Input: part model. Units: mm. Frame: model coordinates. A direction names the side the tool comes from. Give positions to 0.01 mm unless a question says otherwise; leave off trailing zeros. Loops run counter-clockwise (first coordinate to the right, second up) from the corner with the lowest first, then second, coordinate; pieces in that order, holes last. Notation, with made-up numbers: (77, 39.25) -> (103, 39.25) arc R33 ccw to (103, 73.25) -> close; hole circle Ø9 at (24, 42.25). An arc over 180 degrees is marked (long way). Answer in a Markdown table with one row per item. Add a question column.
```python
from build123d import *

# Parameters (mm, degrees)
F0_W     = 32
F0_H     = 55
F3_DEPTH = 5
F1_R     = 1.75
F4_DEPTH = 19
F5_DEPTH = 5
F6_W     = 50
F6_H     = 4
F7_DEPTH = 1.8
F8_R     = 5
F9_R     = 5
F10_R    = 5
F11_R    = 5
F12_R    = 2
F13_R    = 1


with BuildPart() as f3:
    # F0 (on Front) → F3 (new body)
    with BuildSketch(Plane.XZ):
        with Locations((-113.3904078007, -8.5524536016)):
            Rectangle(F0_W, F0_H)
    extrude(amount=F3_DEPTH)

    # F1 (on face) → F4 (join)
    with BuildSketch(Plane.XZ):
        with Locations((-123.8904078007, 12.9475463984)):
            Circle(F1_R)
        with Locations((-102.8904078007, 12.9475463984)):
            Circle(F1_R)
    extrude(amount=F4_DEPTH)

    # F2 (on face) → F5 (cut)
    with BuildSketch(Plane.XZ):
        with BuildLine():
            ThreePointArc((-116.3904078007, -12.0524536016), (-113.3904078007, -15.0524536016), (-110.3904078007, -12.0524536016))
            ThreePointArc((-110.3904078007, -12.0524536016), (-113.3904078007, -9.0524536016), (-116.3904078007, -12.0524536016))
        make_face()
        with BuildLine():
            Line((-110.3904078007, -30.0524536016), (-110.3904078007, -12.0524536016))
            ThreePointArc((-110.3904078007, -12.0524536016), (-113.3904078007, -15.0524536016), (-116.3904078007, -12.0524536016))
            Line((-116.3904078007, -12.0524536016), (-116.3904078007, -30.0524536016))
            ThreePointArc((-116.3904078007, -30.0524536016), (-113.3904078007, -27.0524536016), (-110.3904078007, -30.0524536016))
        make_face()
        with BuildLine():
            ThreePointArc((-116.3904078007, -30.0524536016), (-113.3904078007, -33.0524536016), (-110.3904078007, -30.0524536016))
            ThreePointArc((-110.3904078007, -30.0524536016), (-113.3904078007, -27.0524536016), (-116.3904078007, -30.0524536016))
        make_face()
    extrude(amount=F5_DEPTH, mode=Mode.SUBTRACT)

    # F6 (on Front) → F7 (cut)
    with BuildSketch(Plane.XZ):
        with Locations((-109.2482896921, 6.9475463984)):
            Rectangle(F6_W, F6_H)
    extrude(amount=F7_DEPTH, mode=Mode.SUBTRACT)

    # F8
    f8_edges = [f3.edges().sort_by_distance(p)[0] for p in [
        (-97.390408, -2.5, 18.947546),
    ]]
    fillet(f8_edges, radius=F8_R)

    # F9
    f9_edges = [f3.edges().sort_by_distance(p)[0] for p in [
        (-129.390408, -2.5, 18.947546),
    ]]
    fillet(f9_edges, radius=F9_R)

    # F10
    f10_edges = [f3.edges().sort_by_distance(p)[0] for p in [
        (-129.390408, -2.5, -36.052454),
    ]]
    fillet(f10_edges, radius=F10_R)

    # F11
    f11_edges = [f3.edges().sort_by_distance(p)[0] for p in [
        (-97.390408, -2.5, -36.052454),
    ]]
    fillet(f11_edges, radius=F11_R)

    # F12
    f12_edges = [f3.edges().sort_by_distance(p)[0] for p in [
        (-98.854874, -5, 17.48308),
        (-113.390408, -5, 18.947546),
        (-127.925942, -5, 17.48308),
        (-129.390408, -5, -8.552454),
        (-127.925942, -5, -34.587988),
        (-113.390408, -5, -36.052454),
        (-97.390408, -5, -8.552454),
    ]]
    fillet(f12_edges, radius=F12_R)

    # F13
    f13_edges = [f3.edges().sort_by_distance(p)[0] for p in [
        (-125.640408, -19, 12.947546),
        (-104.640408, -19, 12.947546),
    ]]
    fillet(f13_edges, radius=F13_R)


solid = f3.part
```
1) Pull-direction query (Z, two-part tool) for faces 1 (the face through (-114, -1, 4.948)), 2 (the face through (-101.22, -11.41, 13.47)), 3 (the face through (-127.965, -1.521, -34.549)), 4 (the face through (-127.89, -1.52, 17.52)); classes: +Z half, -Z half, draft (parallel to the pull), parting line (faces both ways), or undercut.
2) Section A-A on z = -19.5. Output: boundary loops of the cut face in (x, y), and give its area (3 significant figures).
3) Section D-D on y = -4. Output: boundary loops of the cut face in (x, z).
4) Material intervals for line 1 along Z through (x, y) = (-112.5, -0.75); line 2 along Y through (x, z) = (-111.5, 3); line 3 along Y through (x, z) = (-107, 5.5), sorted ascending.
5) Section C-C on z = -3.5. Output: boundary loops of the cut face in (x, y).
6) Pin query (flat end, axial travel): pin 1 (8.5 mm diameter, centred on x = -117.5, z = -18.5, fed in from -Y); pin 2 (5 mm diameter, centred on y = -9, z = 8.5, fed in from +X); pin 3 (1.5 mm diameter, centred on x = -123.5, y = -12, fed in from +Z); pin 4 (1 mm diameter, centred on x = -104.5, y = -16.5, fed in from +Z). Return the tip coordinate at first contact, or that it passes through.
7) Reachability of faces 5 (the face through (-114, -1, 8.948)), 6 (the face through (-103, -19, 13)), 7 (the face through (-116.39, -2, -21)) from +Z, -Z, +X, -X, +Y, -Y: full face, straight path, thin tool, end or side. Return the list, or none.
8) Section B-B on x = -117. Output: boundary loops of the cut face in (y, z), and give its area (3 significant figures).
Working result:
| question | item | result |
|---|---|---|
| 1 | face 1 | undercut |
| 1 | face 2 | parting line |
| 1 | face 3 | -Z half |
| 1 | face 4 | +Z half |
| 2 | outline | (-129.39, -3) arc R2 ccw to (-127.39, -5) -> (-116.39, -5) -> (-116.39, 0) -> (-129.39, 0) -> close; (-110.39, -5) -> (-99.39, -5) arc R2 ccw to (-97.39, -3) -> (-97.39, 0) -> (-110.39, 0) -> close |
| 2 | area | 128 mm2 |
| 3 | outline | (-129.12, -31.05) arc R4.73 ccw to (-124.39, -35.78) -> (-102.39, -35.78) arc R4.73 ccw to (-97.66, -31.05) -> (-97.66, 13.95) arc R4.73 ccw to (-102.39, 18.68) -> (-124.39, 18.68) arc R4.73 ccw to (-129.12, 13.95) -> close; hole (-116.39, -30.05) arc R3 ccw to (-110.39, -30.05) -> (-110.39, -12.05) arc R3 ccw to (-116.39, -12.05) -> close |
| 4 | line 1 | z = -36.05 to -32.92, -9.19 to 4.95, 8.95 to 18.95 |
| 4 | line 2 | y = -5 to 0 |
| 4 | line 3 | y = -5 to -1.8 |
| 5 | outline | (-129.39, -3) arc R2 ccw to (-127.39, -5) -> (-99.39, -5) arc R2 ccw to (-97.39, -3) -> (-97.39, 0) -> (-129.39, 0) -> close |
| 6 | pin 1 | stops at y = -5 |
| 6 | pin 2 | passes through |
| 6 | pin 3 | stops at z = 14.7 |
| 6 | pin 4 | stops at z = 14.3 |
| 7 | face 5 | +X, -X, +Y |
| 7 | face 6 | +Z, -Z, +X, -X, -Y |
| 7 | face 7 | +Y, -Y |
| 8 | outline | (-5, -34.05) arc R2 ccw to (-3, -36.05) -> (0, -36.05) -> (0, 4.95) -> (-1.8, 4.95) -> (-1.8, 8.95) -> (0, 8.95) -> (0, 18.95) -> (-3, 18.95) arc R2 ccw to (-5, 16.95) -> close |
| 8 | area | 266 mm2 |
